Could you check a few things on this model? Use its own coordinates, in mm. A direction names the side the tool comes from. Round coordinates to 2 decimals unless told otherwise and drop trailing zeros. Write each loop counter-clockwise with the first axis right and the second up, starting at its lowest first coordinate (ties: lowest second). Pieces come first, ordered by that corner, then holes.
```python
from build123d import *

# Parameters (mm, degrees)
SKETCH1_W                                       = 75
SKETCH1_H                                       = 24
BOSS_EXTRUDE1_DEPTH                             = 24
SKETCH2_W                                       = 20
SKETCH2_H                                       = 12
CUT_EXTRUDE1_DEPTH                              = 24
FILLET1_START                                   = -1
FILLET1_DEPTH                                   = 26
FILLET1_2_DEPTH                                 = 24
CSK_FOR_M4_FLAT_HEAD_MACHINE_SCREW1_D           = 4.5
CSK_FOR_M4_FLAT_HEAD_MACHINE_SCREW1_CSINK_D     = 9.4
CSK_FOR_M4_FLAT_HEAD_MACHINE_SCREW1_CSINK_ANGLE = 90
M10X1_5_TAPPED_HOLE1_D                          = 8.5
M10X1_5_TAPPED_HOLE1_CSINK_D                    = 10.05
M10X1_5_TAPPED_HOLE1_CSINK_ANGLE                = 90


with BuildPart() as part:
    # Sketch1 → Boss-Extrude1 (new body)
    with BuildSketch(Plane(origin=(0, 0, 0), x_dir=(0, 0, -1), z_dir=(1, 0, 0))):
        Rectangle(SKETCH1_W, SKETCH1_H)
    extrude(amount=BOSS_EXTRUDE1_DEPTH)

    # Sketch2 → Cut-Extrude1 (cut)
    with BuildSketch(Plane(origin=(24, 0, 0), x_dir=(0, 0, -1), z_dir=(1, 0, 0))):
        with Locations((-27.5, 6)):
            Rectangle(SKETCH2_W, SKETCH2_H)
    cut_extrude1 = extrude(amount=-CUT_EXTRUDE1_DEPTH, mode=Mode.SUBTRACT)

    # Fillet1: read off the stored shape, not the designer's step
    # Fillet1 outline → Fillet1 (cut)
    with BuildSketch(Plane.YZ.offset(FILLET1_START)):
        with BuildLine():
            Line((12, 17.5), (6, 17.5))
            ThreePointArc((6, 17.5), (10.242640687, 15.742640687), (12, 11.5))
            Line((12, 11.5), (12, 17.5))
        make_face()
    fillet1 = extrude(amount=FILLET1_DEPTH, mode=Mode.SUBTRACT)

    # Fillet1 2 outline → Fillet1 2 (add)
    with BuildSketch(Plane.YZ):
        with BuildLine():
            Line((0, 17.5), (6, 17.5))
            ThreePointArc((6, 17.5), (1.757359313, 19.257359313), (0, 23.5))
            Line((0, 23.5), (0, 17.5))
        make_face()
    fillet1_2 = extrude(amount=FILLET1_2_DEPTH)

    # CSK for M4 Flat Head Machine Screw1 (through all)
    with Locations(Plane(origin=(0, 0, 0), x_dir=(1, 0, 0), z_dir=(0, 1, 0))):
        with Locations((6, -28.5), (18, -28.702489343)):
            csk_for_m4_flat_head_machine_screw1 = CounterSinkHole(CSK_FOR_M4_FLAT_HEAD_MACHINE_SCREW1_D / 2, CSK_FOR_M4_FLAT_HEAD_MACHINE_SCREW1_CSINK_D / 2, counter_sink_angle=CSK_FOR_M4_FLAT_HEAD_MACHINE_SCREW1_CSINK_ANGLE)

    # Mirror1: Cut-Extrude1, Fillet1, Fillet1 2, CSK for M4 Flat Head Machine Screw1 across plane
    add(cut_extrude1.mirror(Plane.XY), mode=Mode.SUBTRACT)
    add(fillet1.mirror(Plane.XY), mode=Mode.SUBTRACT)
    add(fillet1_2.mirror(Plane.XY))
    add(csk_for_m4_flat_head_machine_screw1.mirror(Plane.XY), mode=Mode.SUBTRACT)

    # M10x1.5 Tapped Hole1 (through all)
    with Locations(Plane(origin=(24, 0, 0), x_dir=(0, 0, -1), z_dir=(1, 0, 0))):
        with Locations((0, 0)):
            CounterSinkHole(M10X1_5_TAPPED_HOLE1_D / 2, M10X1_5_TAPPED_HOLE1_CSINK_D / 2, counter_sink_angle=M10X1_5_TAPPED_HOLE1_CSINK_ANGLE)


solid = part.part
```
Q1. On a 3-axis mill with a long thin cutter (end or side, diameter ignored), from which of +Z, -Z, +X, -X, +Y, -Y can I reach the whole of each face in a straight line? I mean faces 1 (the flat face through (12, 12, 0)), 2 (the flat face through (12, 0, 32)), 3 (the flat face through (12, 0, -32)). Say none if no direction works.
Q2. Imagine slicing it at A-A, the plane x = 18. Write out the boundary of the cut face in (y, z), then the cut area to 3 significant figures.
Q3. We'd pull the mould along X, two halves only. Please class faces 4 (the flat face through (12, -12, 1)), 5 (the flat face through (0, -6, -1)), 6 (the cylindrical face through (4.962, -7.292, 30.496)): pulls with the +X half, pulls with the -X half, needs draft (parallel to the pull), parting line crosses it, or undercut.
Q4. If I drill on L1, parallel to X at y = -5.5, z = 28.5; L2, parallel to Z at x = 18, y = -4.5; L3, parallel to Y at x = 11, z = 0, over which ranges is the centre line in solid material (lowest first)?
Q5. I'm going to push flat-ended pins straight in: pin 1 Ø6 at (x, y) = (19, 8.5) entering from -Z; pin 2 Ø4 at (x, z) = (21.5, 21.5) entering from +Y; pin 3 Ø1.5 at (x, z) = (13, 21) entering from +Y. Where does each tip first touch, or does it pass through?
Q6. Imagine slicing it at C-C, the plane y = -9.75. Write out the boundary of the cut face in (x, z), then the cut area to 3 significant figures.
Q7. Imagine slicing it at B-B, the plane z = 0. Write out the boundary of the cut face in (x, y) (3 decimals), then the cut area to 3 significant figures.
Results found:
1. face 1: +Z, -Z, +X, -X, +Y
1. face 2: +Z, +X, -X, +Y
1. face 3: -Z, +X, -X, +Y
2. outline: (-12, -37.5) - (0, -37.5) - (0, -33.4) - (-2.45, -30.95) - (-12, -30.95) - close; (-12, -26.45) - (-2.45, -26.45) - (0, -24) - (0, -23.5) arc R6 cw to (6, -17.5) arc R6 ccw to (12, -11.5) - (12, 11.5) arc R6 ccw to (6, 17.5) arc R6 cw to (0, 23.5) - (0, 24) - (-2.45, 26.45) - (-12, 26.45) - close; (-12, 30.95) - (-2.45, 30.95) - (0, 33.4) - (0, 37.5) - (-12, 37.5) - close; hole circle Ø8.5 at (0, 0)
2. area: 1,140 mm2
3. face 4: needs draft
3. face 5: pulls with the -X half
3. face 6: undercut
4. L1: x = 0 to 3.75, 8.25 to 15.76, 20.24 to 24
4. L2: z = -37.5 to -30.95, -26.45 to 26.45, 30.95 to 37.5
4. L3: y = -12 to -4.25, 4.25 to 12
5. pin 1: stops at z = -17.52
5. pin 2: stops at y = 1.53
5. pin 3: stops at y = 0.96
6. outline: (0, -37.5) - (24, -37.5) - (24, 37.5) - (0, 37.5) - close; hole circle Ø4.5 at (6, -28.5); hole circle Ø4.5 at (6, 28.5); hole circle Ø4.5 at (18, -28.7); hole circle Ø4.5 at (18, 28.7)
6. area: 1,740 mm2
7. outline: (0, -12) - (24, -12) - (24, -5.025) - (23.225, -4.25) - (0, -4.25) - close; (0, 4.25) - (23.225, 4.25) - (24, 5.025) - (24, 12) - (0, 12) - close
7. area: 371 mm2
